from build123d import *

# Parameters (mm, degrees)
SKETCH1_R           = 50
BOSS_EXTRUDE1_DEPTH = 2
SKETCH4_R           = 2
CUT_EXTRUDE1_DEPTH  = 2
SKETCH5_R           = 50
SKETCH5_R_2         = 48
BOSS_EXTRUDE2_DEPTH = 100
SKETCH6_R           = 2
BOSS_EXTRUDE3_DEPTH = 20
SKETCH7_R           = 3.5
CUT_EXTRUDE2_DEPTH  = 5
SKETCH8_R           = 1.45
CUT_EXTRUDE3_DEPTH  = 10


with BuildPart() as part:
    # Sketch1 → Boss-Extrude1 (new body)
    with BuildSketch(Plane(origin=(0, 0, 0), x_dir=(1, 0, 0), z_dir=(0, 1, 0))):
        Circle(SKETCH1_R)
    extrude(amount=BOSS_EXTRUDE1_DEPTH)

    # Sketch4 → Cut-Extrude1 (cut)
    with BuildSketch(Plane(origin=(0, 2, 0), x_dir=(1, 0, 0), z_dir=(0, 1, 0))):
        with Locations((-7.5, 0)):
            Circle(SKETCH4_R)
        with Locations((7.5, 0)):
            Circle(SKETCH4_R)
    extrude(amount=-CUT_EXTRUDE1_DEPTH, mode=Mode.SUBTRACT)

    # Sketch5 → Boss-Extrude2 (add)
    with BuildSketch(Plane(origin=(0, 2, 0), x_dir=(1, 0, 0), z_dir=(0, 1, 0))):
        Circle(SKETCH5_R)
        Circle(SKETCH5_R_2, mode=Mode.SUBTRACT)
    extrude(amount=BOSS_EXTRUDE2_DEPTH)

    # Sketch6 → Boss-Extrude3 (add)
    with BuildSketch(Plane(origin=(0, 2, 0), x_dir=(1, 0, 0), z_dir=(0, 1, 0))):
        Circle(SKETCH6_R)
    extrude(amount=BOSS_EXTRUDE3_DEPTH)

    # Sketch7 → Cut-Extrude2 (cut)
    with BuildSketch(Plane(origin=(0, 2, 0), x_dir=(1, 0, 0), z_dir=(0, 1, 0))):
        with Locations((0, -35)):
            Circle(SKETCH7_R)
    extrude(amount=-CUT_EXTRUDE2_DEPTH, mode=Mode.SUBTRACT)

    # Sketch8 → Cut-Extrude3 (cut)
    with BuildSketch(Plane(origin=(0, 2, 0), x_dir=(1, 0, 0), z_dir=(0, 1, 0))):
        with Locations((0.238867715, -32.008273773)):
            Circle(SKETCH8_R)
        with Locations((-32.724876918, 0.318490286)):
            Circle(SKETCH8_R)
        with Locations((-0.238867715, 32.963744632)):
            Circle(SKETCH8_R)
        with Locations((31.769406059, 0.159245143)):
            Circle(SKETCH8_R)
    extrude(amount=-CUT_EXTRUDE3_DEPTH, mode=Mode.SUBTRACT)


solid = part.part
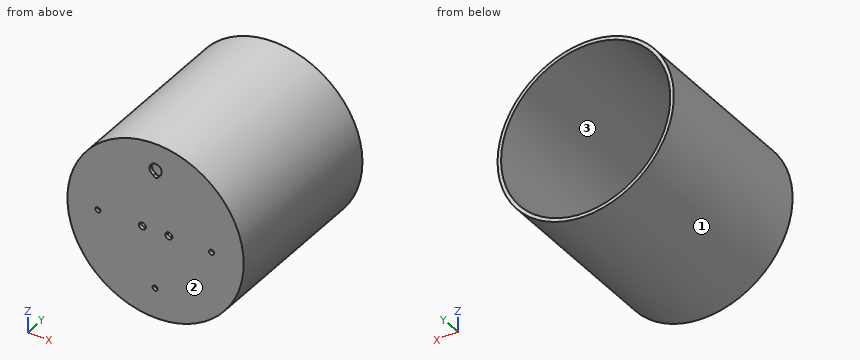
Check sheet for the modelled part. Datum: model origin and axes. Units: mm. Face numbers are marked on the shaded views. Give positions to 0.01 mm unless a question says otherwise; leave off trailing zeros. Write each loop counter-clockwise with the first axis right and the second up, starting at its lowest first coordinate (ties: lowest second). Pieces come first, ordered by that corner, then holes. Notation, with made-up numbers: (41.5, -39) -> (68.5, -39) arc R30 ccw to (68.5, 0) -> close; hole circle Ø11 at (23, 56.25). An arc over 180 degrees is marked (long way). Use one line per item in the form item = value. Start each with the question number.
1. Section check A-A (x = -8). Record the cut outline in (y, z), and give its area (3 significant figures).
2. Section check C-C (y = 44). Record the cut outline in (x, z), and give its area (3 significant figures).
3. Mould release check, pull along X, two halves, no side actions. Record for the marked faces 1, 2 and 3: pulls with the +X half, pulls with the -X half, needs draft (parallel to the pull), parting line crosses it, or undercut.
4. Thickness scan on line 1 along X through (y, z) = (1.3, 0); line 2 along Z through (x, y) = (0, 32); line 3 along X through (y, z) = (32.5, -27). Record the ranges inside material, lowest first. Write a range as from..to.
5. Section check B-B (z = 35.5). Record the cut outline in (x, y), and give its area (3 significant figures).
6. Go/stop test with flat-tipped pins: P1, Ø2, axis at x = -15, y = 49.5, coming from the -Z side; P2, Ø4.5, axis at x = 1, z = 0, coming from the +Y side; P3, Ø12, axis at y = 75, z = 36.5, coming from the -X side; P4, Ø3.5, axis at x = 31.77, z = -0.16, coming from the -Y side. Record where each tip stops, or that it passes through.
7. Section check D-D (z = 8.5). Record the cut outline in (x, y), and give its area (3 significant figures).
Conclusion:
q1.outline = (0, -49.36) -> (102, -49.36) -> (102, -47.33) -> (2, -47.33) -> (2, -1.94) -> (0, -1.94) -> close; (0, 1.94) -> (2, 1.94) -> (2, 47.33) -> (102, 47.33) -> (102, 49.36) -> (0, 49.36) -> close
q1.area = 595 mm²
q2.outline = circle Ø100 at (0, 0); hole circle Ø96 at (0, 0)
q2.area = 616 mm²
q3.face_1 = parting line crosses it
q3.face_2 = needs draft
q3.face_3 = undercut
q4.line_1 = -50..-34.14, -31.31..-9.5, -5.5..5.5, 9.5..30.33, 33.21..50
q4.line_2 = -50..-48, 48..50
q4.line_3 = -42.08..-39.69, 39.69..42.08
q5.outline = (-35.21, 0) -> (-3.46, 0) -> (-3.46, 2) -> (-32.31, 2) -> (-32.31, 102) -> (-35.21, 102) -> close; (3.46, 0) -> (35.21, 0) -> (35.21, 102) -> (32.31, 102) -> (32.31, 2) -> (3.46, 2) -> close
q5.area = 708 mm²
q6.P1 = -48
q6.P2 = 22
q6.P3 = -39.62
q6.P4 = 0
q7.outline = (-49.27, 0) -> (49.27, 0) -> (49.27, 102) -> (47.24, 102) -> (47.24, 2) -> (-47.24, 2) -> (-47.24, 102) -> (-49.27, 102) -> close
q7.area = 603 mm²
